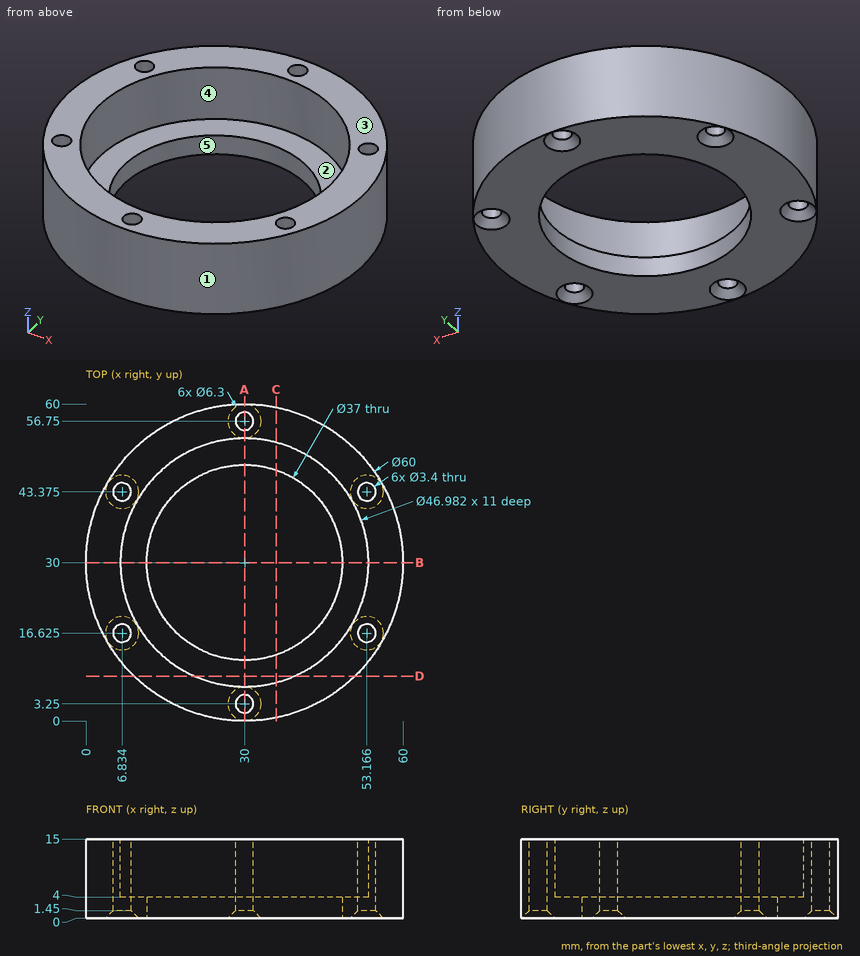
Verification items for this drawing (mm, ordinates from the low corner). A direction names the side the tool comes from. Coordinates: 2 decimals unless noted, no trailing zeros. Order: outer loops, then holes, each group sorted by start corner. A loop starts at its lowest first (then second) coordinate and runs counter-clockwise, first axis right, second up. Notation, with made-up numbers: M 88,79 L 117,79 A27 ccw 117,118 Z; hole C 33.25,-6 d5. An arc over 180 degrees is marked long. Write each question's results on one line, items separated by ' | '.
1) Section check D-D on y = 8.5. Record the cut outline in (x, z) (1 decimal).
Solved:
outline: M 9.1,0 L 50.9,0 L 50.9,15 L 39.5,15 L 39.5,4 L 20.5,4 L 20.5,15 L 9.1,15 Z
2) Section check B-B on y = 30. Record the cut outline in (x, z).
Solved:
outline: M 0,0 L 11.5,0 L 11.5,4 L 6.51,4 L 6.51,15 L 0,15 Z; M 48.5,0 L 60,0 L 60,15 L 53.49,15 L 53.49,4 L 48.5,4 Z
3) Section check C-C on x = 36. Record the cut outline in (y, z).
Solved:
outline: M 0.61,0 L 12.5,0 L 12.5,4 L 7.29,4 L 7.29,15 L 0.61,15 Z; M 47.5,0 L 59.39,0 L 59.39,15 L 52.71,15 L 52.71,4 L 47.5,4 Z
4) Scan lines: line 1 along Y through (x, z) = (30, 2.25); line 2 along Y through (x, z) = (39.5, 10.75) (1 decimal); line 3 along X through (y, z) = (18, 3.5) (1 decimal). Record each from-to range of solid material in increasing order. Write a range as [from, to].
Solved:
line 1: y = [0, 1.55], [4.95, 11.5], [48.5, 55.05], [58.45, 60] | line 2: y = [1.5, 8.5], [51.5, 58.5] | line 3: x = [2.5, 5.8], [7.8, 15.9], [44.1, 52.2], [54.2, 57.5]
5) Release check for a two-part mould opening along X. For the marked faces 1, 2 and 3 record: pulls with the +X half, pulls with the -X half, needs draft (parallel to the pull), parting line crosses it, or undercut.
Solved:
face 1: parting line crosses it | face 2: undercut | face 3: needs draft
6) Gauge pin test, flat ends, axial feed: pin 1 Ø6 at (y, z) = (23, 9) entering from -X; pin 2 Ø1.5 at (y, z) = (52.5, 9.5) entering from +X; pin 3 Ø1.5 at (y, z) = (24.5, 11) entering from -X. Record the tip position at first contact, or that the pin passes through.
Solved:
pin 1: stops at x = 0.27 | pin 2: stops at x = 50.66 | pin 3: stops at x = 0.38
7) Access from +Z, -Z, +X, -X, +Y, -Y to the whole of each face (thin tool, end or side, straight path). Record for the marked faces 4 and 5.
Solved:
face 4: +Z | face 5: +Z, -Z
8) Section check A-A on x = 30. Record the cut outline in (y, z), plus the area to 3 significant figures.
Solved:
outline: M 0,0 L 0.1,0 L 1.55,1.45 L 1.55,15 L 0,15 Z; M 4.95,1.45 L 6.4,0 L 11.5,0 L 11.5,4 L 6.51,4 L 6.51,15 L 4.95,15 Z; M 48.5,0 L 53.6,0 L 55.05,1.45 L 55.05,15 L 53.49,15 L 53.49,4 L 48.5,4 Z; M 58.45,1.45 L 59.9,0 L 60,0 L 60,15 L 58.45,15 Z | area: 129 mm²
